Autodesk Inventor part; units mm, degrees
ref_plane "YZ Plane" through (0, 0, 0) normal (1, 0, 0) x (0, 1, 0)
ref_plane "XZ Plane" through (0, 0, 0) normal (0, 1, 0) x (-1, 0, 0)
ref_plane "XY Plane" through (0, 0, 0) normal (0, 0, 1) x (1, 0, 0)
sketch "Skizze1" plane through (0, 0, 0) normal (0, 1, 0) x (-1, 0, 0)
  line L0 (35, 52.5) -> (-35, 52.5)
  line L1 (-35, 52.5) -> (-35, -52.5)
  line L2 (-35, -52.5) -> (35, -52.5)
  line L3 (35, -52.5) -> (35, 52.5)
  point P0 (0, 0)
  point P1 (0, 52.5)
  point P2 (35, 0)
  dimension "d0" = 105
  dimension "d1" = 70
extrude "Extrusion1" add sketch "Skizze1" along normal blind 48
shell "Wandung1" thickness 2 removed faces 1 at (11.6667, 0, 17.5)
sketch "Skizze25" plane through (0, 0, 0) normal (0, -1, 0) x (1, 0, 0)
  line L0 (33, 50.5) -> (33, -50.5) construction
  line L1 (-33, 50.5) -> (33, 50.5) construction
  line L2 (-33, -50.5) -> (-33, 50.5) construction
  line L3 (33, -50.5) -> (-33, -50.5) construction
  line L4 (33, 50.5) -> (28, 50.5)
  line L5 (28, 50.5) -> (28, 45.5)
  line L6 (28, 45.5) -> (33, 45.5)
  line L7 (33, 45.5) -> (33, 50.5)
  line L8 (33, -50.5) -> (28, -50.5)
  line L9 (28, -50.5) -> (28, -45.5)
  line L10 (28, -45.5) -> (33, -45.5)
  line L11 (33, -45.5) -> (33, -50.5)
  line L12 (-33, 50.5) -> (-28, 50.5)
  line L13 (-28, 50.5) -> (-28, 45.5)
  line L14 (-28, 45.5) -> (-33, 45.5)
  line L15 (-33, 45.5) -> (-33, 50.5)
  line L16 (-33, -50.5) -> (-28, -50.5)
  line L17 (-28, -50.5) -> (-28, -45.5)
  line L18 (-28, -45.5) -> (-33, -45.5)
  line L19 (-33, -45.5) -> (-33, -50.5)
  point P0 (0, 0)
  dimension "d208" = 5
  dimension "d209" = 5
extrude "Extrusion12" add sketch "Skizze25" against normal blind 8
chamfer "Fase2" distance 5 angle 45 2 edges at (30.5, 8, 45.5) (28, 8, 48)
chamfer "Fase3" distance 5 angle 45 2 edges at (30.5, 8, -45.5) (28, 8, -48)
chamfer "Fase4" distance 5 angle 45 2 edges at (-28, 8, 48) (-30.5, 8, 45.5)
chamfer "Fase5" distance 5 angle 45 2 edges at (-28, 8, -48) (-30.5, 8, -45.5)
sketch "Skizze26" plane through (0, 0, 0) normal (0, -1, 0) x (1, 0, 0)
  line L0 (-31, 48.5) -> (31, 48.5) construction
  line L1 (31, 48.5) -> (31, -48.5) construction
  line L2 (31, -48.5) -> (-31, -48.5) construction
  line L3 (-31, -48.5) -> (-31, 48.5) construction
  point P0 (0, 0)
  point P1 (-31, 0)
  point P2 (0, 48.5)
  dimension "d224" = 97
  dimension "d225" = 62
hole "Bohrung14" at (-31, 0, 48.5) at (31, 0, 48.5) at (31, 0, -48.5) at (-31, 0, -48.5) direction (0, 1, 0) diameter 2.8 depth 8
chamfer "Fase6" distance 1 angle 45 8 edges at (0, 48, -52.5) (35, 48, 0) (35, 24, -52.5) (0, 48, 52.5) (35, 24, 52.5) (-35, 24, 52.5) (-35, 48, 0) (-35, 24, -52.5)
sketch "Skizze11" plane through (35, 45, -52.5) normal (1, 0, 0) x (0, 0, 1)
  circle A0 centre (37.5, 33) radius 9 construction
  line L0 (104, 45) -> (1, 45) construction
  point P0 (52.5, 45)
  point P1 (52.5, 45)
  point P2 (52.5, 45)
  dimension "d238" = 18
  dimension "d285" = 15
  dimension "d286" = 12
hole "Button" [suppressed]
sketch "Skizze12" plane through (0, 48, 0) normal (0, 1, 0) x (1, 0, 0)
  point P0 (0, 0)
  point P1 (10, 25)
  point P2 (10, 15)
  point P3 (10, 5)
  dimension "d239" = 5
  dimension "d240" = 10
  dimension "d241" = 10
  dimension "d258" = 10
hole "LEDS" at (10, 48, -25) at (10, 48, -15) at (10, 48, -5) direction (0, -1, 0) diameter 3 end through all
sketch "Skizze14" plane through (29, 0, -52.5) normal (0, 0, -1) x (-1, 0, 0)
  line L0 (-5, 0) -> (63, 0) construction
  point P0 (9, 10)
  point P1 (29, 0)
  point P2 (29, 0)
  point P3 (29, 0)
  point P4 (29, 0)
  dimension "d268" = 10
  dimension "d287" = 20
hole "Sensor" [suppressed]
sketch "Skizze20" plane through (-29, 0, 52.5) normal (0, 0, 1) x (1, 0, 0)
  line L0 (38.5, 17.5) -> (49.5, 17.5)
  line L1 (49.5, 17.5) -> (49.5, 12.5)
  line L2 (49.5, 12.5) -> (38.5, 12.5)
  line L3 (38.5, 12.5) -> (38.5, 17.5)
  line L4 (38.5, 15) -> (49.5, 15) construction
  line L5 (44, 17.5) -> (44, 12.5) construction
  line L6 (-5, 0) -> (63, 0) construction
  point P0 (51.5, 15)
  point P1 (36.5, 15)
  point P2 (44, 15)
  point P3 (29, 0)
  point P4 (29, 0)
  point P5 (29, 0)
  point P6 (44, 15)
  point P7 (29, 0)
  dimension "d149" = 11
  dimension "d150" = 5
  dimension "d153" = 15
  dimension "d249" = 15
  dimension "d259" = 15
extrude "Extrusion9" cut sketch "Skizze20" against normal up to surface (2 mm away)
hole "Switch" at (7.5, 15, 52.5) at (22.5, 15, 52.5) direction (0, 0, -1) diameter 2.5 depth 2
sketch "Skizze22" plane through (35, 0, 52.5) normal (-1, 0, 0) x (0, 0, 1)
  line L0 (-104, 0) -> (-1, 0) construction
  point P0 (-29, 14.5)
  point P1 (-52.5, 0)
  point P2 (-52.5, 0)
  point P3 (-52.5, 0)
  point P4 (0, 0)
  dimension "d250" = 23.5
  dimension "d251" = 14.5
  dimension "d260" = 29
hole "nRF-Antenna" at (35, 14.5, 23.5) direction (-1, 0, 0) diameter 13 depth 8 tip angle 118
sketch "Skizze27" plane through (-33, 46, 50.5) normal (0, -1, 0) x (1, 0, 0)
  line L0 (59, -94) -> (7, -94) construction
  line L1 (7, -94) -> (7, -7) construction
  line L2 (7, -7) -> (59, -7) construction
  line L3 (59, -7) -> (59, -94) construction
  circle A0 centre (59, -94) radius 3.5
  circle A1 centre (7, -94) radius 3.5
  circle A2 centre (7, -7) radius 3.5
  circle A3 centre (59, -7) radius 3.5
  circle A4 centre (59, -94) radius 1.4
  circle A5 centre (7, -94) radius 1.4
  circle A6 centre (59, -7) radius 1.4
  circle A7 centre (7, -7) radius 1.4
  point P0 (33, -50.5)
  point P1 (59, -50.5)
  point P2 (33, -94)
  dimension "d252" = 7
  dimension "d253" = 87
  dimension "d254" = 52
  dimension "d255" = 2.8
extrude "PCB-holder" add sketch "Skizze27" along normal blind 10
sketch "Skizze29" plane through (0, 48, 0) normal (0, 1, 0) x (1, 0, 0)
  point P0 (0, 0)
  point P1 (-8, 15)
  dimension "d269" = 8
  dimension "d278" = 15
hole "LED Green" at (-8, 48, -15) direction (0, -1, 0) diameter 3 depth 8 tip angle 118
sketch "Skizze30" plane through (34, 0, -52.5) normal (0, 0, -1) x (-1, 0, 0)
  line L0 (16.5, 17) -> (31.5, 17)
  line L1 (31.5, 17) -> (31.5, 28)
  line L2 (31.5, 28) -> (16.5, 28)
  line L3 (16.5, 28) -> (16.5, 17)
  line L4 (24, 17) -> (24, 28) construction
  line L5 (16.5, 22.5) -> (31.5, 22.5) construction
  line L6 (0, 0) -> (68, 0) construction
  line L7 (22.5, 48) -> (25.5, 48) construction
  line L8 (22.5, 48) -> (25.5, 48) construction
  line L9 (22.5, 48) -> (25.5, 48) construction
  line L10 (0, 48) -> (68, 48) construction
  line L11 (68, 48) -> (0, 48) construction
  point P0 (34, 0)
  point P1 (34, 0)
  point P2 (24, 22.5)
  point P3 (34, 0)
  point P4 (40.5, 48)
  point P5 (43.5, 48)
  dimension "d279" = 15
  dimension "d280" = 11
  dimension "d282" = 10
  dimension "d288" = 20
extrude "Arduino Programming" [suppressed]
sketch "Skizze31" plane through (-34, 0, 52.5) normal (0, 0, 1) x (1, 0, 0)
  line L0 (17.5, 28) -> (30.5, 28)
  line L1 (30.5, 28) -> (30.5, 38)
  line L2 (30.5, 38) -> (17.5, 38)
  line L3 (17.5, 38) -> (17.5, 28)
  line L4 (24, 28) -> (24, 38) construction
  line L5 (17.5, 33) -> (30.5, 33) construction
  line L6 (0, 0) -> (68, 0) construction
  point P0 (34, 0)
  point P1 (34, 0)
  point P2 (24, 33)
  dimension "d289" = 10
  dimension "d290" = 33
  dimension "d291" = 13
  dimension "d292" = 10
extrude "USB-C" cut sketch "Skizze31" against normal blind 10
sketch "Skizze32" plane through (0, 48, 0) normal (0, 1, 0) x (1, 0, 0)
  line L0 (34, 52.5) -> (-34, 52.5) construction
  point P0 (0, 0)
  point P1 (-5, 40)
  point P2 (-2, 40)
  point P3 (1, 40)
  dimension "d295" = 3
  dimension "d296" = 3
  dimension "d297" = 40
  dimension "d298" = 5
  dimension "d309" = 12.5
hole "Bohrung16" at (-5, 48, -40) at (-2, 48, -40) at (1, 48, -40) direction (0, -1, 0) diameter 1.5 depth 8 tip angle 118
pattern_circular "Runde Anordnung3" count 7 over 360 about axis through (-5, 44, -40) along (0, 1, 0) of "Bohrung16"
equation "\"d209\" = d208"
properties part number "Top_handheld" material "PC/ABS-Kunststoff"
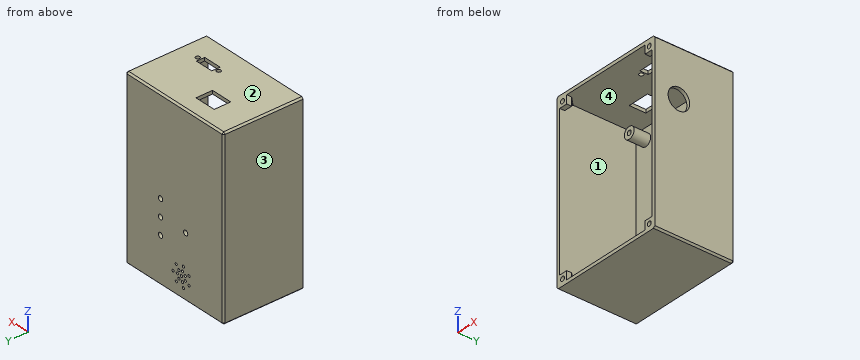
Work out the finished part from the listing and answer in its coordinate system (mm). Face numbers are marked on the shaded views. Give positions to 0.01 mm unless a question says otherwise; leave off trailing zeros. Order: outer loops, then holes, each group sorted by start corner. A loop starts at its lowest first (then second) coordinate and runs counter-clockwise, first axis right, second up. Notation, with made-up numbers: (74.25, -0.5) -> (120.25, -0.5) arc R17 cw to (120.25, 5.5) -> close; hole circle Ø5 at (50.25, -1.5). An arc over 180 degrees is marked (long way). Answer as a JSON object with one key per item and string values. Group by question number.
1. Consider line 1 along X through (y, z) = (15, 51); line 2 along X through (y, z) = (24, 5); line 3 along Z through (x, y) = (31.5, 25). Determine where each line is inside the solid, lowest interval first. Write a range as [from, to].
2. Section A-A on x = 17 is taken. Determine the outline of the cut face in (y, z).
3. The mould has two halves that part along X. Classify the marked faces 1, 2, 3 and 4: released by +X, released by -X, zero draft, split by the parting line, or undercut.
4. Section D-D on x = 26 is taken. Determine the outline of the cut face in (y, z).
5. Section C-C on x = -18 is taken. Determine the outline of the cut face in (y, z), plus the area to 3 significant figures.
6. Section B-B on z = 33 is taken. Determine the outline of the cut face in (x, y), plus the area to 3 significant figures.
7. Flat-ended cylindrical pins translate along their axes: pin 1 Ø0.9 at (x, z) = (-1.26, -44.69) entering from -Y; pin 2 Ø5.5 at (x, z) = (-24.5, 42.5) entering from -Y; pin 3 Ø3 at (x, y) = (7.5, 15) entering from +Z; pin 4 Ø3 at (x, z) = (-25, -30.5) entering from -Y. Find the tip coordinate at first contact, or state that the pin passes through.
Result sheet:
{
 "1": {"line 1": "x = [-35, 6.25], [8.75, 9.5], [20.5, 21.25], [23.75, 35]", "line 2": "x = [-35, -33], [33, 35]", "line 3": "z = [-52.5, -50.5], [50.5, 52.5]"},
 "2": {"outline": "(0, -52.5) -> (47, -52.5) -> (48, -51.5) -> (48, 51.5) -> (47, 52.5) -> (17.5, 52.5) -> (17.5, 50.5) -> (46, 50.5) -> (46, -50.5) -> (0, -50.5) -> close; (0, 50.5) -> (12.5, 50.5) -> (12.5, 52.5) -> (0, 52.5) -> close"},
 "3": {"face 1": "undercut", "face 2": "zero draft", "face 3": "released by -X", "face 4": "undercut"},
 "4": {"outline": "(0, -52.5) -> (47, -52.5) -> (48, -51.5) -> (48, 51.5) -> (47, 52.5) -> (0, 52.5) -> (0, 50.5) -> (46, 50.5) -> (46, 47) -> (36, 47) -> (36, 44.9) -> (46, 44.9) -> (46, 42.1) -> (36, 42.1) -> (36, 40) -> (46, 40) -> (46, -40) -> (36, -40) -> (36, -42.1) -> (46, -42.1) -> (46, -44.9) -> (36, -44.9) -> (36, -47) -> (46, -47) -> (46, -50.5) -> (0, -50.5) -> close"},
 "5": {"outline": "(0, -52.5) -> (47, -52.5) -> (48, -51.5) -> (48, 51.5) -> (47, 52.5) -> (0, 52.5) -> (0, 50.5) -> (46, 50.5) -> (46, -50.5) -> (0, -50.5) -> close", "area": "393 mm^2"},
 "6": {"outline": "(-35, 0) -> (-33, 0) -> (-33, 46) -> (33, 46) -> (33, 0) -> (35, 0) -> (35, 47) -> (34, 48) -> (-34, 48) -> (-35, 47) -> close", "area": "323 mm^2"},
 "7": {"pin 1": "passes through", "pin 2": "stops at y = 36", "pin 3": "stops at z = 52.5", "pin 4": "stops at y = 46"}
}
